```python
from build123d import *

# Parameters (mm, degrees)
ESBO_O1_R                     = 120
RESSALTO_EXTRUS_O1_DEPTH      = 200
RESSALTO_EXTRUS_O1_DEPTH_BACK = 220
CORTE_EXTRUS_O1_REACH         = 422
ESBO_O2_R                     = 112
RESSALTO_EXTRUS_O3_DEPTH      = 3
RESSALTO_EXTRUS_O3_DEPTH_BACK = 3
FILETE2_R                     = 3


with BuildPart() as part:
    # Esbo_o1 → Ressalto-extrus_o1 (new body, two sides)
    with BuildSketch(Plane(origin=(0, 0, 0), x_dir=(1, 0, 0), z_dir=(0, 1, 0))) as ressalto_extrus_o1_sk:
        Circle(ESBO_O1_R)
    extrude(amount=RESSALTO_EXTRUS_O1_DEPTH)
    extrude(ressalto_extrus_o1_sk.sketch, amount=-RESSALTO_EXTRUS_O1_DEPTH_BACK)

    # Esbo_o2 → Corte-extrus_o1 (cut, up to next)
    with BuildSketch(Plane(origin=(0, 200, 0), x_dir=(1, 0, 0), z_dir=(0, 1, 0)), mode=Mode.PRIVATE) as corte_extrus_o1_sk1:
        Circle(ESBO_O2_R)
    corte_extrus_o1_tool1 = extrude(corte_extrus_o1_sk1.sketch, amount=-CORTE_EXTRUS_O1_REACH, mode=Mode.PRIVATE) & part.part
    add(corte_extrus_o1_tool1.solids().sort_by_distance((0, 200, 0))[0], mode=Mode.SUBTRACT)

    # Esbo_o4 → Ressalto-extrus_o3 (add, two sides)
    with BuildSketch(Plane.XY) as ressalto_extrus_o3_sk:
        Polygon((-118.712281772, 320), (-118.712281772, 200), (-112.712281772, 200), (-112.712281772, 314), (113.045365563, 314), (113.045365563, 200), (119.045365563, 200), (119.045365563, 320), align=None)
    extrude(amount=RESSALTO_EXTRUS_O3_DEPTH)
    extrude(ressalto_extrus_o3_sk.sketch, amount=-RESSALTO_EXTRUS_O3_DEPTH_BACK)

    # Filete2
    filete2_edges = [part.edges().sort_by_distance(p)[0] for p in [
        (-118.712281772, 320, 0),
        (119.045365563, 320, 0),
    ]]
    fillet(filete2_edges, radius=FILETE2_R)


solid = part.part
```
Can you work these out from the model? Positions are in its coordinate system, mm. A direction names the side the tool comes from. Round coordinates to 2 decimals unless told otherwise and drop trailing zeros. Loops run counter-clockwise (first coordinate to the right, second up) from the corner with the lowest first, then second, coordinate; pieces in that order, holes last.
Item 1: If we mould it in two halves opening along Z, with no side actions, what happens to faces 3 (the flat face through (79.4, 200, 79.4)), 4 (the cylindrical face through (103.46, -7.06, 42.9)), 5 (the flat face through (0, 318, -3))? For each: +Z half, -Z half, draft (parallel to the pull), parting line (faces both ways), or undercut.
Item 2: Which directions (+Z, -Z, +X, -X, +Y, -Y) give clear straight access to the entire face, cutting with the end or side of a thin tool? Please do faces 1 (the flat face through (79.4, -220, 79.4)), 2 (the flat face through (0, 318, 3)).
Item 3: Suppose I cut it at D-D, the plane y = -26. Write out the boundary of the cut face in (x, z).
Item 4: Please list where these lines run through material, in increasing order: L1, parallel to X at y = 80, z = 0; L2, parallel to X at y = -194.5, z = 28.5.
Item 5: Will these pins go through, and if not, where does the flat tip stop? pin 1 Ø6.5 at (y, z) = (250.5, 1.5) entering from -X; pin 2 Ø1.5 at (x, y) = (68, -147) entering from -Z; pin 3 Ø6.5 at (y, z) = (268.5, -1) entering from +X.
Item 6: Suppose I cut it at B-B, the plane z = 81. Write out the boundary of the cut face in (x, y), then the cut area to 3 significant figures.
Item 7: Suppose I cut it at A-A, the plane y = 257. Write out the boundary of the cut face in (x, z).
Item 8: Suppose I cut it at C-C, the plane x = 0. Write out the boundary of the cut face in (y, z), then the cut area to 3 significant figures.
Reported:
1. face 3: draft
1. face 4: undercut
1. face 5: -Z half
2. face 1: +Z, -Z, +X, -X, -Y
2. face 2: +Z, +X, -X, +Y
3. outline: circle Ø240 at (0, 0); hole circle Ø224 at (0, 0)
4. L1: x = -120 to -112, 112 to 120
4. L2: x = -116.57 to -108.31, 108.31 to 116.57
5. pin 1: stops at x = -118.71
5. pin 2: stops at z = -99.39
5. pin 3: stops at x = 119.05
6. outline: (-88.54, -220) - (-77.35, -220) - (-77.35, 200) - (-88.54, 200) - close; (77.35, -220) - (88.54, -220) - (88.54, 200) - (77.35, 200) - close
6. area: 9,400 mm2
7. outline: (-118.71, -3) - (-112.71, -3) - (-112.71, 3) - (-118.71, 3) - close; (113.05, -3) - (119.05, -3) - (119.05, 3) - (113.05, 3) - close
8. outline: (-220, -120) - (200, -120) - (200, -112) - (-220, -112) - close; (-220, 112) - (200, 112) - (200, 120) - (-220, 120) - close; (314, -3) - (320, -3) - (320, 3) - (314, 3) - close
8. area: 6,760 mm2
